Autodesk Inventor part; units mm, degrees
ref_plane "YZ Plane" through (0, 0, 0) normal (1, 0, 0) x (0, 1, 0)
ref_plane "XZ Plane" through (0, 0, 0) normal (0, 1, 0) x (-1, 0, 0)
ref_plane "XY Plane" through (0, 0, 0) normal (0, 0, 1) x (1, 0, 0)
sketch "Sketch1" plane through (0, 0, 0) normal (0, 0, 1) x (1, 0, 0)
  line L0 (8.35, -7) -> (8.35, -9) construction
  line L1 (8.35, -9) -> (7.35, -9) construction
  line L2 (7.35, -9) -> (7.35, -7) construction
  line L3 (7.35, -7) -> (8.35, -7) construction
  line L4 (9.45, -5.5) -> (9.45, -7.5) construction
  line L5 (9.45, -7.5) -> (8.45, -7.5) construction
  line L6 (8.45, -7.5) -> (8.45, -5.5) construction
  line L7 (8.45, -5.5) -> (9.45, -5.5) construction
  line L8 (2.45, 4.2) -> (2.45, -4.2) construction
  line L9 (2.45, -4.2) -> (-5.95, -4.2) construction
  line L10 (-5.95, -4.2) -> (-5.95, 4.2) construction
  line L11 (-5.95, 4.2) -> (2.45, 4.2) construction
  circle A0 centre (-2.6, 10.5) radius 1 construction
  circle A1 centre (9.9, 10.5) radius 1 construction
  circle A2 centre (-2.6, -10.5) radius 1 construction
  circle A3 centre (9.9, -10.5) radius 1 construction
  line L12 (11.95, 12.5) -> (-11.95, 12.5)
  line L13 (-11.95, 12.5) -> (-11.95, -12.5)
  line L14 (-11.95, -12.5) -> (11.95, -12.5)
  line L15 (11.95, -12.5) -> (11.95, 12.5) construction
  line L16 (5.7177, -12.5) -> (14.5315, -12.5) construction
  line L17 (11.95, -4.2) -> (9.45, -4.2)
  line L18 (-5.95, -4.2) -> (-5.95, 4.2)
  line L19 (-5.95, 4.2) -> (11.95, 4.2)
  line L20 (7.35, -4.2) -> (7.35, -9)
  line L21 (7.35, -9) -> (9.45, -9)
  line L22 (9.45, -9) -> (9.45, -4.2)
  line L23 (7.35, -4.2) -> (-5.95, -4.2)
  circle A4 centre (-2.6, -10.5) radius 0.9
  circle A5 centre (9.9, -10.5) radius 0.9
  circle A6 centre (9.9, 10.5) radius 0.9
  circle A7 centre (-2.6, 10.5) radius 0.9
  line L24 (23.45, 23.5) -> (23.45, -23.5)
  line L25 (-23.55, 23.5) -> (23.45, 23.5)
  line L26 (-23.55, 12.5) -> (-23.55, 23.5)
  line L27 (-23.55, 12.5) -> (-11.95, 12.5)
  line L28 (-11.95, -12.5) -> (-23.55, -12.5)
  line L29 (-23.55, -23.5) -> (-23.55, -12.5)
  line L30 (23.45, -23.5) -> (-23.55, -23.5)
  line L31 (11.95, 4.2) -> (11.95, -4.2)
  line L32 (-23.55, 12.5) -> (-23.55, -12.5)
  circle A8 centre (-18.05, 18) radius 1.4
  circle A9 centre (17.95, 18) radius 1.4
  circle A10 centre (17.95, -18) radius 1.4
  circle A11 centre (-18.05, -18) radius 1.4
  point P0 (0, 0)
  dimension "d4" = 1.8
  dimension "d5" = 1.8
  dimension "d6" = 1.8
  dimension "d7" = 1.8
extrude "Extrusion1" add sketch "Sketch1" along normal blind 3
Input: part model. Units: mm. Frame: model coordinates. A direction names the side the tool comes from. Round coordinates to 2 decimals unless told otherwise and drop trailing zeros. Loops run counter-clockwise (first coordinate to the right, second up) from the corner with the lowest first, then second, coordinate; pieces in that order, holes last. Notation, with made-up numbers: (-35, 48.5) -> (-27, 48.5) arc R17 ccw to (-27, 75.5) -> close; hole circle Ø10 at (23, -39.75). An arc over 180 degrees is marked (long way). Use one line per item in the form item = value. Start each with the question number.
Item 1: Material intervals for L1, parallel to Y at x = 17.95, z = 0.95; L2, parallel to Y at x = 8, z = 1.8; L3, parallel to X at y = -18.5, z = 2.65, sorted ascending. Write a range as from..to.
Item 2: Section query B-B on x = 0. Return the cut outline in (y, z).
Item 3: Section query C-C on y = -18. Return the cut outline in (x, z).
Item 4: Contact query for a flat-ended pin moving along its axis: pin 1 Ø1.6 at (x, y) = (-2.6, -10.5) entering from +Z. Output: stop coordinate, or through.
Item 5: Section query A-A on y = -1.5. Return the cut outline in (x, z).
Item 6: Section query D-D on x = -18.05. Return the cut outline in (y, z), then the cut area to 3 significant figures.
Item 7: Set-up query: faces 5 (the face through (0, 6, 3)), 6 (the face through (8, -9, 1)). Return all of +Z, -Z, +X, -X, +Y, -Y with unobstructed straight access to the full face (end or side cutting, diameter ignored); none if empty.
Item 8: Mould query, pull axis Y, two halves, no side actions, for faces 1 (the face through (11, -4.2, 1)), 2 (the face through (3, 4.2, 1)), 3 (the face through (0, -23.5, 1)), 4 (the face through (23.45, 0, 1)). Classes: pulls with the +Y half, pulls with the -Y half, needs draft (parallel to the pull), parting line crosses it, or undercut.
Ans:
q1.L1 = -23.5..-19.4, -16.6..16.6, 19.4..23.5
q1.L2 = -23.5..-9, 4.2..23.5
q1.L3 = -23.55..-19.36, -16.74..16.64, 19.26..23.45
q2.outline = (-23.5, 0) -> (-4.2, 0) -> (-4.2, 3) -> (-23.5, 3) -> close; (4.2, 0) -> (23.5, 0) -> (23.5, 3) -> (4.2, 3) -> close
q3.outline = (-23.55, 0) -> (-19.45, 0) -> (-19.45, 3) -> (-23.55, 3) -> close; (-16.65, 0) -> (16.55, 0) -> (16.55, 3) -> (-16.65, 3) -> close; (19.35, 0) -> (23.45, 0) -> (23.45, 3) -> (19.35, 3) -> close
q4.pin_1 = through
q5.outline = (-23.55, 0) -> (-5.95, 0) -> (-5.95, 3) -> (-23.55, 3) -> close; (11.95, 0) -> (23.45, 0) -> (23.45, 3) -> (11.95, 3) -> close
q6.outline = (-23.5, 0) -> (-19.4, 0) -> (-19.4, 3) -> (-23.5, 3) -> close; (-16.6, 0) -> (16.6, 0) -> (16.6, 3) -> (-16.6, 3) -> close; (19.4, 0) -> (23.5, 0) -> (23.5, 3) -> (19.4, 3) -> close
q6.area = 124 mm^2
q7.face_5 = +Z, +X, -X, +Y, -Y
q7.face_6 = +Z, -Z
q8.face_1 = undercut
q8.face_2 = undercut
q8.face_3 = pulls with the -Y half
q8.face_4 = needs draft
